from build123d import *

# Parameters (mm, degrees)
F0_W      = 70
F0_H      = 20
F1_DEPTH  = 6.5
F4_DEPTH  = 4
F5_R      = 2.6
F6_DEPTH  = 13.001
F7_DEPTH  = 13.001
F8_W      = 14
F8_H      = 1.4
F9_DEPTH  = 20.001
F11_R     = 5
F10_R     = 3.1
F12_DEPTH = 20.001
F13_R     = 4.25
F14_DEPTH = 3.5
F16_DEPTH = 5


with BuildPart() as f1:
    # F0 (on Top) → F1 (new body, symmetric)
    with BuildSketch(Plane.XY):
        Rectangle(F0_W, F0_H)
    extrude(amount=F1_DEPTH, both=True)

    # F3 (on face) → F4 (cut)
    with BuildSketch(Plane.XY.offset(6.5)):
        Polygon((-31, -4.6188021535), (-27, -2.3094010768), (-27, 2.3094010768), (-31, 4.6188021535), (-35, 2.3094010768), (-35, -2.3094010768), align=None)
        Polygon((35, -2.3094010768), (35, 2.3094010768), (31, 4.6188021535), (27, 2.3094010768), (27, -2.3094010768), (31, -4.6188021535), align=None)
    extrude(amount=-F4_DEPTH, mode=Mode.SUBTRACT)

    # F5 (on face) → F6 (cut, through all)
    with BuildSketch(Plane.XY.offset(6.5)):
        with Locations((-31, 0)):
            Circle(F5_R)
        with Locations((31, 0)):
            Circle(F5_R)
    extrude(amount=-F6_DEPTH, mode=Mode.SUBTRACT)

    # F2 (on face) → F7 (cut, through all)
    with BuildSketch(Plane.XY.offset(6.5)):
        with BuildLine():
            Line((-15, -3), (15, -3))
            ThreePointArc((15, -3), (18, 0), (15, 3))
            Line((15, 3), (-15, 3))
            ThreePointArc((-15, 3), (-18, 0), (-15, -3))
        make_face()
    extrude(amount=-F7_DEPTH, mode=Mode.SUBTRACT)

    # F8 (on face) → F9 (cut, through all)
    with BuildSketch(Plane.XZ.offset(10)):
        with Locations((-28, -0.2)):
            Rectangle(F8_W, F8_H)
        with Locations((28, -0.2)):
            Rectangle(F8_W, F8_H)
    extrude(amount=-F9_DEPTH, mode=Mode.SUBTRACT)

    # F11
    f11_edges = [f1.edges().sort_by_distance(p)[0] for p in [
        (35, 10, 3.5),
        (35, 10, -3.7),
        (35, -10, 3.5),
        (35, -10, -3.7),
        (-35, -10, -3.7),
        (-35, -10, 3.5),
        (-35, 10, 3.5),
        (-35, 10, -3.7),
    ]]
    fillet(f11_edges, radius=F11_R)

    # F10 (on face) → F12 (cut, through all)
    with BuildSketch(Plane.XZ.offset(10)):
        with Locations((-25.5, -0.5)):
            Circle(F10_R)
        with Locations((25.5, -0.5)):
            Circle(F10_R)
    extrude(amount=-F12_DEPTH, mode=Mode.SUBTRACT)

    # F13 (on face) → F14 (cut)
    with BuildSketch(Plane(origin=(0, 0, -6.5), x_dir=(1, 0, 0), z_dir=(0, 0, -1))):
        with Locations((31, 0)):
            Circle(F13_R)
        with Locations((-31, 0)):
            Circle(F13_R)
    extrude(amount=-F14_DEPTH, mode=Mode.SUBTRACT)

    # F15 (on face) → F16 (cut)
    with BuildSketch(Plane.XY.offset(6.5)):
        Polygon((-17.8867513459, -5), (-12.1132486541, -5), (-9.2264973081, 0), (-12.1132486541, 5), (-17.8867513459, 5), (-20.7735026919, 0), align=None)
        Polygon((-9.2264973081, 0), (-12.1132486541, -5), (12.1132486541, -5), (9.2264973081, 0), (12.1132486541, 5), (-12.1132486541, 5), align=None)
        Polygon((9.2264973081, 0), (12.1132486541, -5), (17.8867513459, -5), (20.7735026919, 0), (17.8867513459, 5), (12.1132486541, 5), align=None)
    extrude(amount=-F16_DEPTH, mode=Mode.SUBTRACT)


solid = f1.part
Design review of the part built by this model. Coordinates are the model's own, in mm. A direction names the side the tool comes from. Give positions to 0.01 mm unless a question says otherwise; leave off trailing zeros. Order: outer loops, then holes, each group sorted by start corner. A loop starts at its lowest first (then second) coordinate and runs counter-clockwise, first axis right, second up. Notation, with made-up numbers: (61.25, -38.5) - (76.25, -38.5) arc R23 cw to (76.25, -12.5) - close; hole circle Ø7 at (-32, -37). An arc over 180 degrees is marked (long way). Use CSV: the item, a comma, the result in double quotes. Start each with the question number.
Q1. Machinability: for faces 5 (the face through (-19.31, 2.535, 4.035)), 6 (the face through (22, 0, -0.9)), 7 (the face through (18, 0, -2)), 8 (the face through (-26.753, 0.166, -4.774)), which of the approach directions +Z, -Z, +X, -X, +Y, -Y give a long, thin tool a straight path to every point of the face, cutting with its end or side? Answer none if there is none.
Q2. Take a section at C-C (y = -9). State the section outline as (x, z) points.
Q3. Draft analysis for pull direction Y (two halves, no side actions). For faces 1 (the face through (33, -9, -4)), 2 (the face through (34, 0, -0.9)), 3 (the face through (33, 9, -4)), 4 (the face through (33, -2, -3)), state which applies: pulls with the +Y half, pulls with the -Y half, needs draft (parallel to the pull), parting line crosses it, or undercut.
Q4. For line 1 (X direction, y = 0, z = -5.35); line 2 (Y direction, x = 6, z = 0.25); line 3 (Y direction, x = -11.5, z = 5.5), list the stretches that pass through material, from the lowest coordinate up.
Q5. Take a section at A-A (x = -13.5). State the section outline as (y, z) points, and give its area (3 significant figures).
Q6. For P1, Ø1.2, axis at y = -0.5, z = 3.5, coming from the -X side; P2, Ø1.5, axis at x = 7.5, y = -2.5, coming from the +Z side; P3, Ø0.7, axis at y = -2, z = 0, coming from the +X side, all flat-tipped, find the tip position at first contact; note any pin that passes through.
Q7. Take a section at B-B (z = 4.25). State the section outline as (x, y) points.
Calculated:
1,face 5,"+Z"
1,face 6,"+X, +Y, -Y"
1,face 7,"+Z, -Z"
1,face 8,"-Z"
2,outline,"(-33, -6.5) - (33, -6.5) - (33, -0.9) - (28.57, -0.9) arc R3.1 cw to (22.43, -0.9) - (21, -0.9) - (21, 0.5) - (22.57, 0.5) arc R3.1 cw to (28.43, 0.5) - (33, 0.5) - (33, 6.5) - (-33, 6.5) - (-33, 0.5) - (-28.43, 0.5) arc R3.1 cw to (-22.57, 0.5) - (-21, 0.5) - (-21, -0.9) - (-22.43, -0.9) arc R3.1 cw to (-28.57, -0.9) - (-33, -0.9) - close"
3,face 1,"pulls with the -Y half"
3,face 2,"needs draft"
3,face 3,"pulls with the +Y half"
3,face 4,"undercut"
4,line 1,"x = -26.75 to -18, 18 to 26.75"
4,line 2,"y = -10 to -3, 3 to 10"
4,line 3,"y = -10 to -5, 5 to 10"
5,outline,"(-10, -6.5) - (-3, -6.5) - (-3, 1.5) - (-5, 1.5) - (-5, 6.5) - (-10, 6.5) - close; (3, -6.5) - (10, -6.5) - (10, 6.5) - (5, 6.5) - (5, 1.5) - (3, 1.5) - close"
5,area,"162 mm²"
6,P1,"stops at x = -27"
6,P2,"stops at z = 1.5"
6,P3,"stops at x = 21"
7,outline,"(-35, -5) arc R5 ccw to (-30, -10) - (30, -10) arc R5 ccw to (35, -5) - (35, -2.31) - (31, -4.62) - (27, -2.31) - (27, 2.31) - (31, 4.62) - (35, 2.31) - (35, 5) arc R5 ccw to (30, 10) - (-30, 10) arc R5 ccw to (-35, 5) - (-35, 2.31) - (-31, 4.62) - (-27, 2.31) - (-27, -2.31) - (-31, -4.62) - (-35, -2.31) - close; hole (-20.77, 0) - (-17.89, -5) - (17.89, -5) - (20.77, 0) - (17.89, 5) - (-17.89, 5) - close"
